```python
from build123d import *

# Parameters (mm, degrees)
SKETCH030_W     = 40
SKETCH030_H     = 40
PAD022_DEPTH    = 1500
SKETCH031_W     = 40
SKETCH031_H     = 40
POCKET008_DEPTH = 20
SKETCH032_W     = 40
SKETCH032_H     = 40
POCKET009_DEPTH = 20
SKETCH059_R     = 5
POCKET014_DEPTH = 40.001


with BuildPart() as part:
    # Sketch030 → Pad022 (new body)
    with BuildSketch(Plane.YZ):
        with Locations((-300, 280)):
            Rectangle(SKETCH030_W, SKETCH030_H)
    extrude(amount=PAD022_DEPTH)

    # Sketch031 (on Face3 of Pad022) → Pocket008 (cut)
    with BuildSketch(Plane.YX.offset(-260)):
        with Locations((-300, 1480)):
            Rectangle(SKETCH031_W, SKETCH031_H)
        with Locations((-300, 920)):
            Rectangle(SKETCH031_W, SKETCH031_H)
        with Locations((-300, 20)):
            Rectangle(SKETCH031_W, SKETCH031_H)
    extrude(amount=-POCKET008_DEPTH, mode=Mode.SUBTRACT)

    # Sketch032 (on Face1 of Pocket008) → Pocket009 (cut)
    with BuildSketch(Plane(origin=(0, 0, 300), x_dir=(0, -1, 0), z_dir=(0, 0, 1))):
        with Locations((300, 1200)):
            Rectangle(SKETCH032_W, SKETCH032_H)
    extrude(amount=-POCKET009_DEPTH, mode=Mode.SUBTRACT)

    # Sketch059 (on Face1 of Pocket009) → Pocket014 (cut, through all)
    with BuildSketch(Plane(origin=(0, 0, 300), x_dir=(0, -1, 0), z_dir=(0, 0, 1))):
        with Locations((300, 20)):
            Circle(SKETCH059_R)
        with Locations((300, 920)):
            Circle(SKETCH059_R)
        with Locations((300, 1480)):
            Circle(SKETCH059_R)
        with Locations((300, 1200)):
            Circle(SKETCH059_R)
    extrude(amount=-POCKET014_DEPTH, mode=Mode.SUBTRACT)


with BuildPart() as part_1:
    # Clone010 placement: moved
    add(part.part.moved(Location((0, 0, 450))))


solid = part_1.part
```
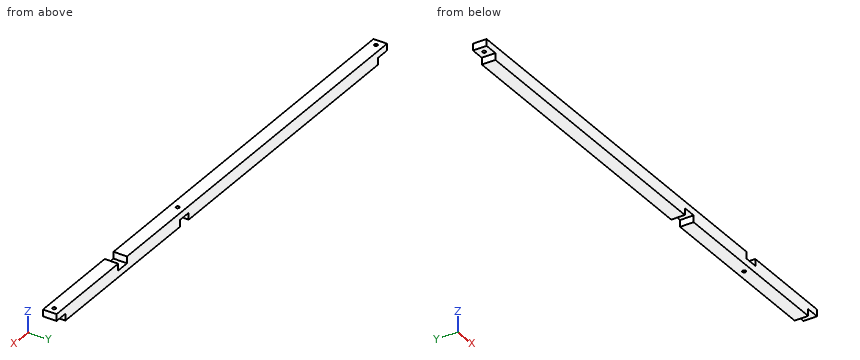
The model under review builds one solid part; all positions refer to its coordinate system, in mm. Give positions to 0.01 mm unless a question says otherwise; leave off trailing zeros. Loops run counter-clockwise (first coordinate to the right, second up) from the corner with the lowest first, then second, coordinate; pieces in that order, holes last. Notation, with made-up numbers: (-34, 14) - (-15, 14) arc R27 ccw to (-15, 37) - close; hole circle Ø9 at (11.25, -39). An arc over 180 degrees is marked (long way). Answer as a JSON object with one key per item and string values.
Q1. Add section B-B on y = -288.5. State the section outline as (x, z) points.
Worked out:
{"outline": "(0, 730) - (40, 730) - (40, 710) - (900, 710) - (900, 730) - (940, 730) - (940, 710) - (1460, 710) - (1460, 730) - (1500, 730) - (1500, 750) - (1220, 750) - (1220, 730) - (1180, 730) - (1180, 750) - (0, 750) - close"}
Q2. Insertion check: pin 1 (12 mm diameter, centred on y = -297.5, z = 728.5, fed in from -X); pin 2 (10 mm diameter, centred on y = -306, z = 717, fed in from -X); pin 3 (8 mm diameter, centred on x = 20, y = -300, fed in from +Z); pin 4 (22 mm diameter, centred on y = -306, z = 717.5, fed in from +X). Each pin has a flat end and moves straight along its axis. Give the tip position at first contact, or say it passes through.
Worked out:
{"pin 1": "stops at x = 0", "pin 2": "stops at x = 40", "pin 3": "passes through", "pin 4": "stops at x = 1460"}
Q3. Add section A-A on z = 717.5. State the section outline as (x, y) points, plus the area to 3 significant figures.
Worked out:
{"outline": "(40, -320) - (900, -320) - (900, -280) - (40, -280) - close; (940, -320) - (1460, -320) - (1460, -280) - (940, -280) - close; hole circle Ø10 at (1200, -300)", "area": "55,100 mm^2"}
Q4. To check wall thickness, follow line 1 along X through (y, z) = (-300, 716); line 2 along Y through (x, z) = (920, 736.75); line 3 along X through (y, z) = (-300, 744). State the ranges of each line that lie inside material, in increasing order.
Worked out:
{"line 1": "x = 40 to 900, 940 to 1195, 1205 to 1460", "line 2": "y = -320 to -305, -295 to -280", "line 3": "x = 0 to 15, 25 to 915, 925 to 1180, 1220 to 1475, 1485 to 1500"}
